from build123d import *

# Parameters (mm, degrees)
SKETCH1_R           = 20
BOSS_EXTRUDE1_DEPTH = 5
SKETCH2_R           = 2
CUT_EXTRUDE1_DEPTH  = 29.722813233
SKETCH3_R           = 9
BOSS_EXTRUDE2_DEPTH = 15
CUT_EXTRUDE2_DEPTH  = 35.641016151
SKETCH5_W           = 1
SKETCH5_H           = 13
CUT_EXTRUDE3_DEPTH  = 12
CUT_EXTRUDE4_REACH  = 42.509
SKETCH7_W           = 17.986100378
SKETCH7_H           = 1
SKETCH8_R           = 3
CUT_EXTRUDE5_DEPTH  = 6
SKETCH9_R           = 2
CUT_EXTRUDE6_DEPTH  = 37.455452322
CHAMFER3_SIZE       = 3
CHAMFER4_SIZE       = 1


with BuildPart() as part:
    # Sketch1 → Boss-Extrude1 (new body)
    with BuildSketch(Plane(origin=(0, 0, 0), x_dir=(1, 0, 0), z_dir=(0, 1, 0))):
        with Locations(Location((0, 0, 0), (0, 0, 270))):
            Circle(SKETCH1_R)
    extrude(amount=BOSS_EXTRUDE1_DEPTH)

    # Sketch2 → Cut-Extrude1 (cut, through all)
    with BuildSketch(Plane(origin=(0, 5, 0), x_dir=(1, 0, 0), z_dir=(0, 1, 0))):
        with Locations(Location((0, 15, 0), (0, 0, 270))):
            Circle(SKETCH2_R)
        with Locations(Location((10.606601718, 10.606601718, 0), (0, 0, 270))):
            Circle(SKETCH2_R)
        with Locations(Location((15, 0, 0), (0, 0, 270))):
            Circle(SKETCH2_R)
        with Locations(Location((10.606601718, -10.606601718, 0), (0, 0, 270))):
            Circle(SKETCH2_R)
        with Locations(Location((0, -15, 0), (0, 0, 270))):
            Circle(SKETCH2_R)
        with Locations(Location((-10.606601718, -10.606601718, 0), (0, 0, 270))):
            Circle(SKETCH2_R)
        with Locations(Location((-15, 0, 0), (0, 0, 270))):
            Circle(SKETCH2_R)
        with Locations(Location((-10.606601718, 10.606601718, 0), (0, 0, 270))):
            Circle(SKETCH2_R)
    extrude(amount=-CUT_EXTRUDE1_DEPTH, mode=Mode.SUBTRACT)

    # Sketch3 → Boss-Extrude2 (add)
    with BuildSketch(Plane(origin=(0, 5, 0), x_dir=(1, 0, 0), z_dir=(0, 1, 0))):
        with Locations(Location((0, 0, 0), (0, 0, 270))):
            Circle(SKETCH3_R)
    extrude(amount=BOSS_EXTRUDE2_DEPTH)

    # Sketch4 → Cut-Extrude2 (cut, through all)
    with BuildSketch(Plane(origin=(0, 20, 0), x_dir=(1, 0, 0), z_dir=(0, 1, 0))):
        with BuildLine():
            Line((1.658312395, 2.5), (-1.658312395, 2.5))
            ThreePointArc((-1.658312395, 2.5), (-1.418637165, -2.643382037), (3, 0))
            ThreePointArc((3, 0), (2.643382037, 1.418637165), (1.658312395, 2.5))
        make_face()
    extrude(amount=-CUT_EXTRUDE2_DEPTH, mode=Mode.SUBTRACT)

    # Sketch5 → Cut-Extrude3 (cut)
    with BuildSketch(Plane(origin=(0, 20, 0), x_dir=(1, 0, 0), z_dir=(0, 1, 0))):
        with Locations((0, -2.5)):
            Rectangle(SKETCH5_W, SKETCH5_H)
    extrude(amount=-CUT_EXTRUDE3_DEPTH, mode=Mode.SUBTRACT)

    # Cut-Extrude4: up to this face of the body (flat: up to its plane)
    cut_extrude4_end = Plane(part.part.faces().sort_by_distance((-0.5, 14, 5.972070135))[0])
    # Sketch7 → Cut-Extrude4 (cut, up to the picked face)
    with BuildSketch(Plane(origin=(9, 0, 0), x_dir=(0, 0, -1), z_dir=(1, 0, 0)), mode=Mode.PRIVATE) as cut_extrude4_sk1:
        with Locations((0.006949811, 8.5)):
            Rectangle(SKETCH7_W, SKETCH7_H)
    cut_extrude4_tool1 = split(extrude(cut_extrude4_sk1.sketch, amount=-CUT_EXTRUDE4_REACH, mode=Mode.PRIVATE), bisect_by=cut_extrude4_end, keep=Keep.BOTH, mode=Mode.PRIVATE)
    add(cut_extrude4_tool1.solids().sort_by(Axis((9, 8.5, -0.00695), (-1, 0, 0)))[0], mode=Mode.SUBTRACT)

    # Sketch8 → Cut-Extrude5 (cut)
    with BuildSketch(Plane(origin=(9, 0, 0), x_dir=(0, 0, -1), z_dir=(1, 0, 0))):
        with Locations((-5.986100378, 14.5)):
            Circle(SKETCH8_R)
        with BuildLine():
            ThreePointArc((-8.986100378, 14.5), (-8.107420721, 16.621320344), (-5.986100378, 17.5))
            Line((-5.986100378, 17.5), (-8.986100378, 17.5))
            Line((-8.986100378, 17.5), (-8.986100378, 14.5))
        make_face()
        with BuildLine():
            ThreePointArc((-5.986100378, 11.5), (-8.107420721, 12.378679656), (-8.986100378, 14.5))
            Line((-8.986100378, 14.5), (-8.986100378, 11.5))
            Line((-8.986100378, 11.5), (-5.986100378, 11.5))
        make_face()
    cut_extrude5 = extrude(amount=-CUT_EXTRUDE5_DEPTH, mode=Mode.SUBTRACT)

    # Mirror1: Cut-Extrude5 across plane
    add(cut_extrude5.mirror(Plane(origin=(0, 0, 0), x_dir=(0, 0, 1), z_dir=(1, 0, 0))), mode=Mode.SUBTRACT)

    # Sketch9 → Cut-Extrude6 (cut, through all)
    with BuildSketch(Plane(origin=(3, 0, 0), x_dir=(0, 0, -1), z_dir=(1, 0, 0))):
        with Locations(Location((-5.986100378, 14.5, 0), (0, 0, 180))):
            Circle(SKETCH9_R)
    extrude(amount=-CUT_EXTRUDE6_DEPTH, mode=Mode.SUBTRACT)

    # Chamfer3
    chamfer3_edges = [part.edges().sort_by_distance(p)[0] for p in [
        (0, 5, -9),
    ]]
    chamfer(chamfer3_edges, length=CHAMFER3_SIZE - 0.0001)  # a hair under: the kernel refuses the full size

    # Chamfer4
    chamfer4_edges = [part.edges().sort_by_distance(p)[0] for p in [
        (0, 5, -20),
    ]]
    chamfer(chamfer4_edges, length=CHAMFER4_SIZE)


solid = part.part
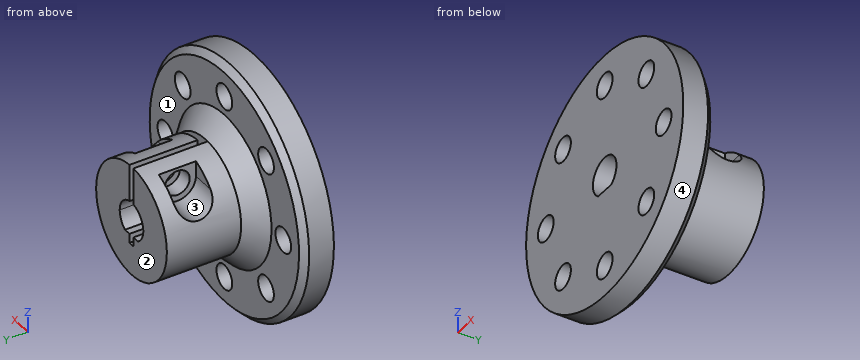
The listing builds one solid part. Answer for the finished solid, in the listing's coordinates (mm). Face numbers are marked on the shaded views. A direction names the side the tool comes from. Give positions to 0.01 mm unless a question says otherwise; leave off trailing zeros. Order: outer loops, then holes, each group sorted by start corner. A loop starts at its lowest first (then second) coordinate and runs counter-clockwise, first axis right, second up. Notation, with made-up numbers: (3.25, 80.5) - (23.25, 80.5) arc R22 cw to (23.25, 111.5) - close; hole circle Ø4 at (52.25, -13). An arc over 180 degrees is marked (long way). Use one line per item in the form item = value.
1) Find section C-C on z = 11. Give the number of separate pieces and of enclosed holes in the cut face, and give its area (3 significant figures).
Verdict:
separate_pieces = 3
enclosed_holes = 0
area = 133 mm^2
2) Consider probe 1 along Y at (x, z) = (5.5, -4); probe 2 along X at (y, z) = (3.25, -9); probe 3 along Y at (x, z) = (9.5, 12.5). Determine where each line is inside the solid, lowest interval first. Write a range as [from, to].
Verdict:
probe_1 = [0, 8], [9, 20]
probe_2 = [-17.86, -11.8], [-9.42, 9.42], [11.8, 17.86]
probe_3 = [0, 5]
3) Find section A-A on y = 14.5. Determine the outline of the cut face in (x, z), and give its area (3 significant figures).
Verdict:
outline = (-8.49, 2.99) arc R9 ccw (long way) to (8.49, 2.99) - (3, 2.99) - (3, 3.99) - (0.5, 3.99) - (0.5, 2.96) arc R3 cw to (1.66, -2.5) - (0.5, -2.5) - (0.5, -4) - (-0.5, -4) - (-0.5, -2.5) - (-1.66, -2.5) arc R3 cw to (-0.5, 2.96) - (-0.5, 3.99) - (-3, 3.99) - (-3, 2.99) - close; (-3, 7.99) - (-0.5, 7.99) - (-0.5, 8.99) arc R9 ccw to (-3, 8.49) - close; (0.5, 7.99) - (3, 7.99) - (3, 8.49) arc R9 ccw to (0.5, 8.99) - close
area = 160 mm^2
4) The mould has two halves that part along X. Classify the marked faces 3 and 4: released by +X, released by -X, zero draft, split by the parting line, or undercut.
Verdict:
face_3 = zero draft
face_4 = split by the parting line
5) For the marked faces 1 and 2, determine the directions among +Z, -Z, +X, -X, +Y, -Y from which every point of the face is accessible in a straight line to the end or side of a thin tool.
Verdict:
face_1 = +Y
face_2 = +Z, -Z, +X, -X, +Y
6) Each of these flat-tipped pins is pushed along its axis until it touches: pin 1 (1 mm diameter, centred on y = 12, z = -0.5, fed in from +X); pin 2 (1.5 mm diameter, centred on x = -14.5, z = 11.5, fed in from -Y); pin 3 (6 mm diameter, centred on x = 8, y = 8.5, fed in from +Z); pin 4 (3.5 mm diameter, centred on x = 10.61, z = 10.61, fed in from +Y). Where does it stop, or does it pass through?
Verdict:
pin_1 = 9
pin_2 = 0
pin_3 = 9
pin_4 = through
7) Find section B-B on y = 18.5. Determine the outline of the cut face in (x, z).
Verdict:
outline = (-1.66, -2.5) arc R3 cw to (-0.5, 2.96) - (-0.5, 8.99) arc R9 ccw (long way) to (0.5, 8.99) - (0.5, 2.96) arc R3 cw to (1.66, -2.5) - (0.5, -2.5) - (0.5, -4) - (-0.5, -4) - (-0.5, -2.5) - close
